Check sheet for the modelled part. Datum: model origin and axes. Units: mm. A direction names the side the tool comes from. Round coordinates to 2 decimals unless told otherwise and drop trailing zeros. Loops run counter-clockwise (first coordinate to the right, second up) from the corner with the lowest first, then second, coordinate; pieces in that order, holes last. Notation, with made-up numbers: (3.5, -28) -> (52.5, -28) arc R24 ccw to (52.5, 5) -> close; hole circle Ø5 at (14, 9). An arc over 180 degrees is marked (long way). Use one line per item in the form item = value. Start each with the question number.
(1) Sectioned sample at C-C (y = 6.35). Record the cut outline in (x, z) (3 decimals).
(2) Material ranges on probe 1 along Y at (x, z) = (0, 28.75) (3 decimals); probe 2 along X at (y, z) = (6.5, 19); probe 3 along Z at (x, y) = (0.75, 6.5), recorded low to high. Write a range as [from, to].
(3) Sectioned sample at A-A (z = 10.25). Record the cut outline in (x, y) (3 decimals).
(4) Set-up check for faces 1 (the cylindrical face through (1.707, 9.027, 17.675)), 2 (the flat face through (6.35, 5, 15)): record each of +Z, -Z, +X, -X, +Y, -Y from which the full face is reachable in a straight line by a thin tool's end or side.
(5) Sectioned sample at D-D (x = -4.5). Record the cut outline in (y, z), and give its area (3 significant figures).
(6) Draft check along X on faces 3 (the cylindrical face through (-5.45, 11.84, 14.79)), 4 (the flat face through (0, 6, 0)), 5 (the cylindrical face through (5.49, 11.8, 14.79)), 6 (the flat face through (0, 6, 5)). Enter one of: released by +X, released by -X, zero draft, split by the parting line, or undercut.
(7) Sectioned sample at B-B (x = 0). Record the cut outline in (y, z) (3 decimals).
(8) Go/stop test with a flat-tipped pin: pin 1 (5.5 mm diameter, centred on x = 0, y = 6.35, fed in from +Z). Record where the tip stops, or that it passes through.
from build123d import *

# Parameters (mm, degrees)
PAD_DEPTH    = 30
SKETCH001_R  = 3.175
POCKET_DEPTH = 25


with BuildPart() as part:
    # Sketch → Pad (new body)
    with BuildSketch(Plane.XY):
        with BuildLine():
            Line((-6.35, 0), (6.35, 0))
            Line((6.35, 0), (6.35, 9.7))
            ThreePointArc((6.35, 9.7), (5.47132, 11.82132), (3.35, 12.7))
            Line((3.35, 12.7), (-3.35, 12.7))
            ThreePointArc((-3.35, 12.7), (-5.47132, 11.82132), (-6.35, 9.7))
            Line((-6.35, 9.7), (-6.35, 0))
        make_face()
    extrude(amount=PAD_DEPTH)

    # Sketch001 (on Face8 of Pad) → Pocket (cut)
    with BuildSketch(Plane.XY.offset(30)):
        with Locations((0, 6.35)):
            Circle(SKETCH001_R)
    extrude(amount=-POCKET_DEPTH, mode=Mode.SUBTRACT)


solid = part.part
Checks:
q1.outline = (-6.35, 0) -> (6.35, 0) -> (6.35, 30) -> (3.175, 30) -> (3.175, 5) -> (-3.175, 5) -> (-3.175, 30) -> (-6.35, 30) -> close
q2.probe_1 = [0, 3.175], [9.525, 12.7]
q2.probe_2 = [-6.35, -3.17], [3.17, 6.35]
q2.probe_3 = [0, 5]
q3.outline = (-6.35, 0) -> (6.35, 0) -> (6.35, 9.7) arc R3 ccw to (3.35, 12.7) -> (-3.35, 12.7) arc R3 ccw to (-6.35, 9.7) -> close; hole circle Ø6.35 at (0, 6.35)
q4.face_1 = +Z
q4.face_2 = +Z, -Z, +X, +Y, -Y
q5.outline = (0, 0) -> (12.47, 0) -> (12.47, 30) -> (0, 30) -> close
q5.area = 374 mm2
q6.face_3 = released by -X
q6.face_4 = zero draft
q6.face_5 = released by +X
q6.face_6 = undercut
q7.outline = (0, 0) -> (12.7, 0) -> (12.7, 30) -> (9.525, 30) -> (9.525, 5) -> (3.175, 5) -> (3.175, 30) -> (0, 30) -> close
q8.pin_1 = 5
